from build123d import *

# Parameters (mm, degrees)
SALIENTE_EXTRUIR1_DEPTH = 2
CROQUIS3_W              = 0.8
CROQUIS3_H              = 3
SALIENTE_EXTRUIR2_DEPTH = 2
CROQUIS4_R              = 0.6
CORTAR_EXTRUIR1_DEPTH   = 44.289721644
CROQUIS5_R              = 1.1
CORTAR_EXTRUIR2_DEPTH   = 44.370496884


with BuildPart() as part:
    # Croquis1 → Saliente-Extruir1 (new body)
    with BuildSketch(Plane.XY):
        Polygon((0, 0), (16, 0), (16, -2), (19, -2), (43, -2), (43, 1), (18, 1), (18, 4), (15, 4), (0, 4), align=None)
    extrude(amount=SALIENTE_EXTRUIR1_DEPTH)

    # Croquis3 → Saliente-Extruir2 (add)
    with BuildSketch(Plane.XY.offset(2)):
        with Locations((42.6, -0.5)):
            Rectangle(CROQUIS3_W, CROQUIS3_H)
    extrude(amount=SALIENTE_EXTRUIR2_DEPTH)

    # Croquis4 → Cortar-Extruir1 (cut, through all)
    with BuildSketch(Plane(origin=(0, 1, 0), x_dir=(1, 0, 0), z_dir=(0, 1, 0))):
        with Locations((39.2, -2)):
            Circle(CROQUIS4_R)
        with Locations((36.2, -2)):
            Circle(CROQUIS4_R)
    extrude(amount=-CORTAR_EXTRUIR1_DEPTH, mode=Mode.SUBTRACT)

    # Croquis5 → Cortar-Extruir2 (cut, through all)
    with BuildSketch(Plane(origin=(0, 0, 0), x_dir=(-1, 0, 0), z_dir=(0, 0, -1))):
        with Locations((-1.5, 2)):
            Circle(CROQUIS5_R)
    extrude(amount=-CORTAR_EXTRUIR2_DEPTH, mode=Mode.SUBTRACT)


solid = part.part
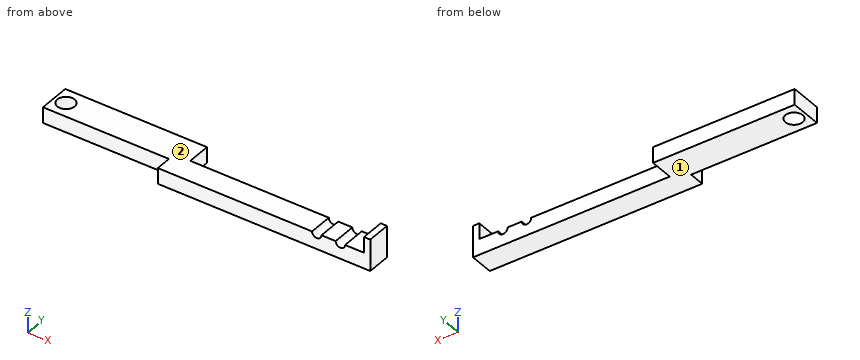
Input: part model. Units: mm. Frame: model coordinates. Face numbers are marked on the shaded views. A direction names the side the tool comes from. Give positions to 0.01 mm unless a question says otherwise; leave off trailing zeros. Write each loop counter-clockwise with the first axis right and the second up, starting at its lowest first coordinate (ties: lowest second). Pieces come first, ordered by that corner, then holes.
Q1. Set-up query: the marked faces 1 and 2. Return all of +Z, -Z, +X, -X, +Y, -Y with unobstructed straight access to the full face (end or side cutting, diameter ignored); none if empty.
Q2. Section D-D, the plane x = 40.5. Output: boundary loops of the cut face in (y, z).
Q3. First-contact query: P1, Ø2, axis at x = 38, y = 0, coming from the +Z side; P2, Ø2, axis at x = 25, z = 2.5, coming from the +Y side; P3, Ø1.8, axis at x = 1.5, y = 2, coming from the -Z side; P4, Ø2, axis at y = 3, z = 1, coming from the +X side. Flat tips, straight axial feed; report the tip coordinate or a pass-through.
Q4. Section C-C, the plane y = -1.6. Output: boundary loops of the cut face in (x, z), plus the area to 3 significant figures.
Q5. Material intervals for probe 1 along Y at (x, z) = (1.5, 0.7); probe 2 along X at (y, z) = (-0.4, 2.6); probe 3 along Y at (x, z) = (13.5, 1.5), sorted ascending.
Q6. Section A-A, the plane z = 0.5. Output: boundary loops of the cut face in (x, y).
Q7. Section B-B, the plane y = 2. Output: boundary loops of the cut face in (x, z).
Filled in:
1. face 1: -Z, +X, -X, +Y, -Y
1. face 2: +Z, -X, +Y, -Y
2. outline: (-2, 0) - (1, 0) - (1, 2) - (-2, 2) - close
3. P1: stops at z = 2
3. P2: stops at y = 1
3. P3: passes through
3. P4: stops at x = 18
4. outline: (16, 0) - (43, 0) - (43, 4) - (42.2, 4) - (42.2, 2) - (39.8, 2) arc R0.6 cw to (38.6, 2) - (36.8, 2) arc R0.6 cw to (35.6, 2) - (16, 2) - close
4. area: 54.5 mm2
5. probe 1: y = 0 to 0.9, 3.1 to 4
5. probe 2: x = 42.2 to 43
5. probe 3: y = 0 to 4
6. outline: (0, 0) - (16, 0) - (16, -2) - (43, -2) - (43, 1) - (18, 1) - (18, 4) - (0, 4) - close; hole circle Ø2.2 at (1.5, 2)
7. outline: (0, 0) - (0.4, 0) - (0.4, 2) - (0, 2) - close; (2.6, 0) - (18, 0) - (18, 2) - (2.6, 2) - close
